```python
from build123d import *

# Parameters (mm, degrees)
SKETCH1_R           = 4.000000001
BOSS_EXTRUDE1_DEPTH = 58.42
CUT_EXTRUDE1_DEPTH  = 10.16
CUT_EXTRUDE5_DEPTH  = 8.89
CUT_EXTRUDE3_START  = -16.423386
SKETCH4_OUTSIDE_W   = 21.902
SKETCH4_OUTSIDE_H   = 21.902
SKETCH4_OUTSIDE_R   = 3.683
CUT_EXTRUDE3_DEPTH  = 1.016
CUT_EXTRUDE4_START  = -5.94995
SKETCH5_OUTSIDE_W   = 21.902
SKETCH5_OUTSIDE_H   = 21.902
SKETCH5_OUTSIDE_R   = 3.683
CUT_EXTRUDE4_DEPTH  = 1.016


with BuildPart() as part:
    # Sketch1 → Boss-Extrude1 (new body)
    with BuildSketch(Plane.XY):
        Circle(SKETCH1_R)
    extrude(amount=BOSS_EXTRUDE1_DEPTH)

    # Sketch2 → Cut-Extrude1 (cut)
    with BuildSketch(Plane.XY.offset(58.42)):
        with BuildLine():
            Line((3.090048545, 2.54), (3.090048545, -2.54))
            ThreePointArc((3.090048545, -2.54), (4.000000001, 0), (3.090048545, 2.54))
        make_face()
    extrude(amount=-CUT_EXTRUDE1_DEPTH, mode=Mode.SUBTRACT)

    # Sketch6 → Cut-Extrude5 (cut)
    with BuildSketch(Plane(origin=(0, 0, 0), x_dir=(-1, 0, 0), z_dir=(0, 0, -1))):
        with BuildLine():
            Line((-3.090048545, 2.54), (-3.090048545, -2.54))
            ThreePointArc((-3.090048545, -2.54), (-4.000000001, 0), (-3.090048545, 2.54))
        make_face()
    extrude(amount=-CUT_EXTRUDE5_DEPTH, mode=Mode.SUBTRACT)

    # Sketch4 outside → Cut-Extrude3 (cut)
    with BuildSketch(Plane(origin=(0, 0, 0), x_dir=(-1, 0, 0), z_dir=(0, 0, -1)).offset(CUT_EXTRUDE3_START)):
        Rectangle(SKETCH4_OUTSIDE_W, SKETCH4_OUTSIDE_H)
        Circle(SKETCH4_OUTSIDE_R, mode=Mode.SUBTRACT)
    extrude(amount=-CUT_EXTRUDE3_DEPTH, mode=Mode.SUBTRACT)

    # Sketch5 outside → Cut-Extrude4 (cut)
    with BuildSketch(Plane.XY.offset(58.42).offset(CUT_EXTRUDE4_START)):
        Rectangle(SKETCH5_OUTSIDE_W, SKETCH5_OUTSIDE_H)
        Circle(SKETCH5_OUTSIDE_R, mode=Mode.SUBTRACT)
    extrude(amount=-CUT_EXTRUDE4_DEPTH, mode=Mode.SUBTRACT)


solid = part.part
```
The listing builds one solid part. Answer for the finished solid, in the listing's coordinates (mm). A direction names the side the tool comes from. Give positions to 0.01 mm unless a question says otherwise; leave off trailing zeros. Order: outer loops, then holes, each group sorted by start corner. A loop starts at its lowest first (then second) coordinate and runs counter-clockwise, first axis right, second up. Notation, with made-up numbers: (-32, -24.75) -> (-15, -24.75) arc R19 cw to (-15, -11.75) -> close; hole circle Ø9 at (17.5, 3.25). An arc over 180 degrees is marked (long way). Answer as CSV lines item,"result". Start each with the question number.
Q1. A cutting plane is placed at B-B (x = 1.5). Determine the outline of the cut face in (y, z).
Q2. Determine the mould class of faces 5 (the flat face through (-1, 0, 58.42)), 6 (the flat face through (3.09, 0, 53)), 7 (the cylindrical face through (-3.68, 0.13, 51.97)) for opening direction Z: pulls with the +Z half, pulls with the -Z half, needs draft (parallel to the pull), parting line crosses it, or undercut.
Q3. A cutting plane is placed at A-A (y = 0). Determine the outline of the cut face in (x, z).
Q4. A cutting plane is placed at D-D (z = 4). Determine the outline of the cut face in (x, y).
Q5. Given pin 1 (3 mm diameter, centred on x = -2.5, z = 44, fed in from -Y); pin 2 (2 mm diameter, centred on x = -2.5, z = 31.5, fed in from +Y); pin 3 (0.5 mm diameter, centred on x = 3.5, y = 0, fed in from -Z), each flat-ended and moving along its own axis, determine where each tip first touches the part or whether it passes through.
Q6. Which of the six approach directions +Z, -Z, +X, -X, +Y, -Y give full straight-line access (tool end or side, diameter ignored) to faces 1 (the flat face through (3.4, 0, 48.26)), 2 (the cylindrical face through (-1.699, -3.267, 16.924)), 3 (the flat face through (-1, 0, 0)), 4 (the flat face through (3.09, 0, 4))?
Q7. Find the intervals of material crossed by L1, parallel to Z at x = -3, y = -2.5; L2, parallel to X at y = 0.25, z = 37.5; L3, parallel to Z at x = 3.75, y = 0.25, in increasing order.
Q8. A cutting plane is placed at C-C (z = 18.5). Determine the outline of the cut face in (x, y), then the cut area to 3 significant figures.
Results found:
1,outline,"(-3.71, 0) -> (3.71, 0) -> (3.71, 16.42) -> (3.36, 16.42) -> (3.36, 17.44) -> (3.71, 17.44) -> (3.71, 51.45) -> (3.36, 51.45) -> (3.36, 52.47) -> (3.71, 52.47) -> (3.71, 58.42) -> (-3.71, 58.42) -> (-3.71, 52.47) -> (-3.36, 52.47) -> (-3.36, 51.45) -> (-3.71, 51.45) -> (-3.71, 17.44) -> (-3.36, 17.44) -> (-3.36, 16.42) -> (-3.71, 16.42) -> close"
2,face 5,"pulls with the +Z half"
2,face 6,"needs draft"
2,face 7,"undercut"
3,outline,"(-4, 0) -> (3.09, 0) -> (3.09, 8.89) -> (4, 8.89) -> (4, 16.42) -> (3.68, 16.42) -> (3.68, 17.44) -> (4, 17.44) -> (4, 48.26) -> (3.09, 48.26) -> (3.09, 58.42) -> (-4, 58.42) -> (-4, 52.47) -> (-3.68, 52.47) -> (-3.68, 51.45) -> (-4, 51.45) -> (-4, 17.44) -> (-3.68, 17.44) -> (-3.68, 16.42) -> (-4, 16.42) -> close"
4,outline,"(3.09, -2.54) -> (3.09, 2.54) arc R4 ccw (long way) to start"
5,pin 1,"y = -3.87"
5,pin 2,"y = 3.71"
5,pin 3,"z = 8.89"
6,face 1,"+Z, +X, +Y, -Y"
6,face 2,"none"
6,face 3,"-Z, +X, -X, +Y, -Y"
6,face 4,"-Z, +X, +Y, -Y"
7,L1,"0 to 16.42, 17.44 to 51.45, 52.47 to 58.42"
7,L2,"-3.99 to 3.99"
7,L3,"8.89 to 16.42, 17.44 to 48.26"
8,outline,"circle Ø8 at (0, 0)"
8,area,"50.3 mm2"
